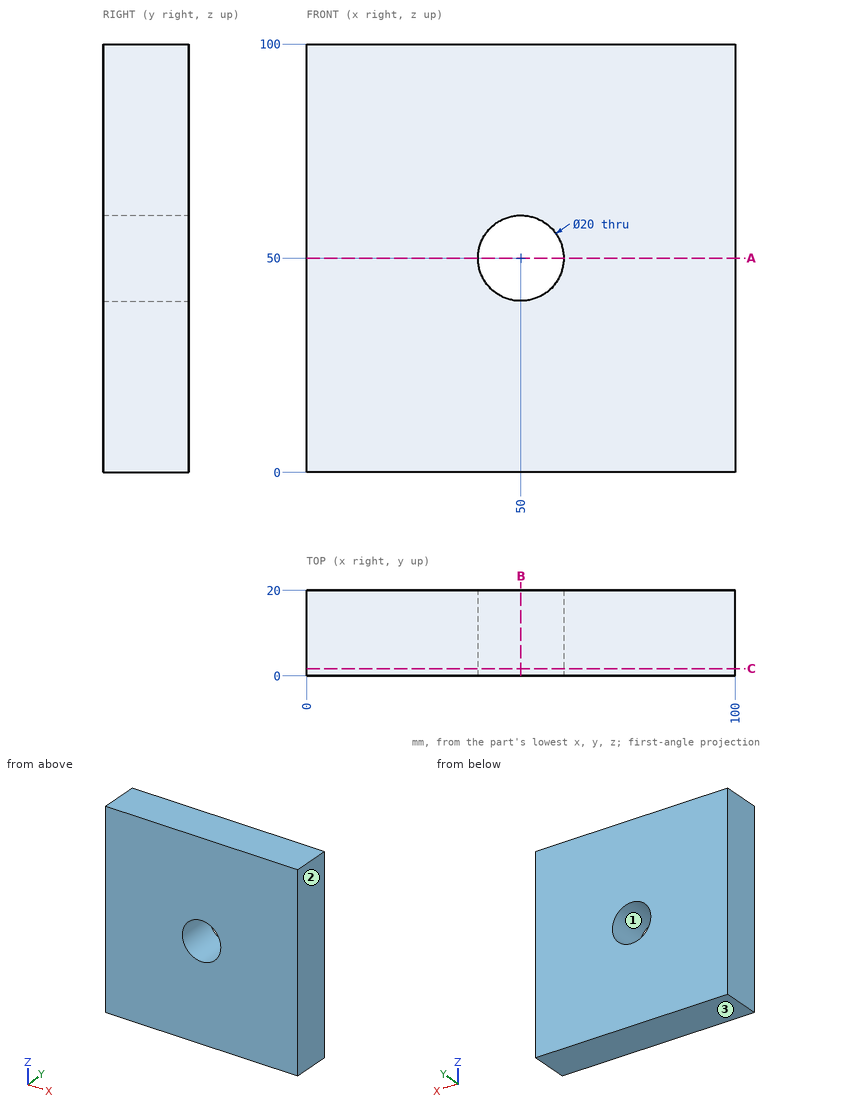
For this review, use the dimensioned drawing (mm, ordinates from the lowest corner) and the shaded views. Round coordinates to 2 decimals unless told otherwise and drop trailing zeros. Loops run counter-clockwise (first coordinate to the right, second up) from the corner with the lowest first, then second, coordinate; pieces in that order, holes last. Notation, with made-up numbers: M 50,40 L 82,40 A26 cw 82,66 Z; hole C -31.75,74.25 d9. An arc over 180 degrees is marked long. Answer as a JSON object with one key per item and string values.
(1) Take a section at B-B on x = 50. Give the boundary of the cut face in (y, z).
Resolved:
{"outline": "M 0,0 L 20,0 L 20,40 L 0,40 Z; M 0,60 L 20,60 L 20,100 L 0,100 Z"}
(2) Take a section at A-A on z = 50. Give the boundary of the cut face in (x, y).
Resolved:
{"outline": "M 0,0 L 40,0 L 40,20 L 0,20 Z; M 60,0 L 100,0 L 100,20 L 60,20 Z"}
(3) Take a section at C-C on y = 1.75. Give the boundary of the cut face in (x, z), and give its area (3 significant figures).
Resolved:
{"outline": "M 0,0 L 100,0 L 100,100 L 0,100 Z; hole C 50,50 d20", "area": "9,690 mm²"}
(4) To check wall thickness, follow line 1 along X through (y, z) = (9, 50); line 2 along Z through (x, y) = (58.5, 4.75). State the ranges of each line that lie inside material, in increasing order.
Resolved:
{"line 1": "0 to 40, 60 to 100", "line 2": "0 to 44.73, 55.27 to 100"}
(5) Clearance check with a flat-ended pin moving along its axis: P1, Ø12, axis at y = 7.5, z = 56.5, coming from the -X side. State where the tip first meets the part, or that it passes through.
Resolved:
{"P1": "x = 0"}
(6) Draft analysis for pull direction Z (two halves, no side actions). For the marked faces 1, 2 and 3, state which applies: released by +Z, released by -Z, zero draft, split by the parting line, or undercut.
Resolved:
{"face 1": "undercut", "face 2": "zero draft", "face 3": "released by -Z"}
